Here's the drawing with two shaded views (mm, measured from the low corner). I have some questions. A direction names the side the tool comes from. Round coordinates to 2 decimals unless told otherwise and drop trailing zeros. Order: outer loops, then holes, each group sorted by start corner. A loop starts at its lowest first (then second) coordinate and runs counter-clockwise, first axis right, second up.
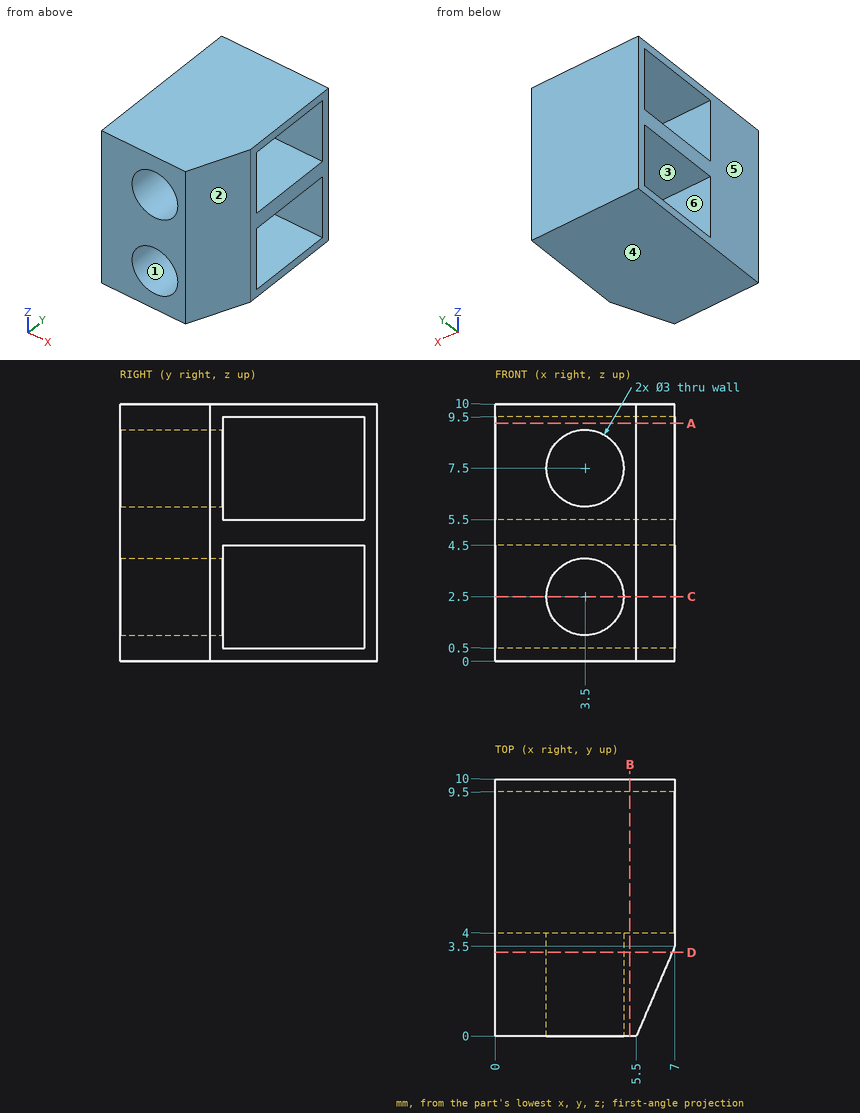
1. If we section it at A-A, the plane z = 9.25: Write out the boundary of the cut face in (x, y), and give its area (3 significant figures).
Evaluation:
outline: (0, 0) - (5.5, 0) - (7, 3.5) - (7, 4) - (0, 4) - close; (0, 9.5) - (7, 9.5) - (7, 10) - (0, 10) - close
area: 28.9 mm2
2. If we section it at D-D, the plane y = 3.25: Write out the boundary of the cut face in (x, z), and give its area (3 significant figures).
Evaluation:
outline: (0, 0) - (6.89, 0) - (6.89, 10) - (0, 10) - close; hole circle Ø3 at (3.5, 2.5); hole circle Ø3 at (3.5, 7.5)
area: 54.8 mm2
3. On a 3-axis mill with a long thin cutter (end or side, diameter ignored), from which of +Z, -Z, +X, -X, +Y, -Y can I reach the whole of each face in a straight line? I mean the marked faces 1, 2 and 3. Say none if no direction works.
Evaluation:
face 1: -Y
face 2: +Z, -Z, +X, -Y
face 3: +X, -X
4. If we section it at B-B, the plane x = 5.25: Write out the boundary of the cut face in (y, z), and give its area (3 significant figures).
Evaluation:
outline: (0, 0) - (10, 0) - (10, 10) - (0, 10) - close; hole (4, 0.5) - (9.5, 0.5) - (9.5, 4.5) - (4, 4.5) - close; hole (4, 5.5) - (9.5, 5.5) - (9.5, 9.5) - (4, 9.5) - close
area: 56.0 mm2
5. If we mould it in two halves opening along Z, with no side actions, what happens to the marked faces 4, 5 and 6? For each: released by +Z, released by -Z, zero draft, split by the parting line, or undercut.
Evaluation:
face 4: released by -Z
face 5: zero draft
face 6: undercut
6. I'm going to push flat-ended pins straight in: P1, Ø3, axis at y = 1.5, z = 2, coming from the +X side; P2, Ø1.8, axis at x = 3.5, z = 7.5, coming from the -Y side; P3, Ø1, axis at y = 6, z = 3, coming from the -X side. Where does each tip first touch, or does it pass through?
Evaluation:
P1: stops at x = 6.79
P2: stops at y = 9.5
P3: passes through
7. I need wall thicknesses on probe 1 along Z at (x, y) = (3.5, 1.1); probe 2 along Z at (x, y) = (3.75, 5.75); probe 3 along Y at (x, z) = (1.75, 2.25). Which ranges of each line are inside material? Lowest first, please.
Evaluation:
probe 1: z = 0 to 1, 4 to 6, 9 to 10
probe 2: z = 0 to 0.5, 4.5 to 5.5, 9.5 to 10
probe 3: y = 0 to 4, 9.5 to 10
8. If we section it at C-C, the plane z = 2.5: Write out the boundary of the cut face in (x, y).
Evaluation:
outline: (0, 0) - (2, 0) - (2, 4) - (0, 4) - close; (0, 9.5) - (7, 9.5) - (7, 10) - (0, 10) - close; (5, 0) - (5.5, 0) - (7, 3.5) - (7, 4) - (5, 4) - close
